Geometry: see drawing. Coordinates: mm, zero at the bounding-box minimum. Coordinates: 2 decimals unless noted, no trailing zeros. Order: outer loops, then holes, each group sorted by start corner. A loop starts at its lowest first (then second) coordinate and runs counter-clockwise, first axis right, second up. Notation, with made-up numbers: (37.5, -29.5) - (45.5, -29.5) arc R22 ccw to (45.5, -14.5) - close; hole circle Ø3 at (30.5, 15.25). An arc over 180 degrees is marked (long way). Use a Markdown table: item, result. Add a question column.
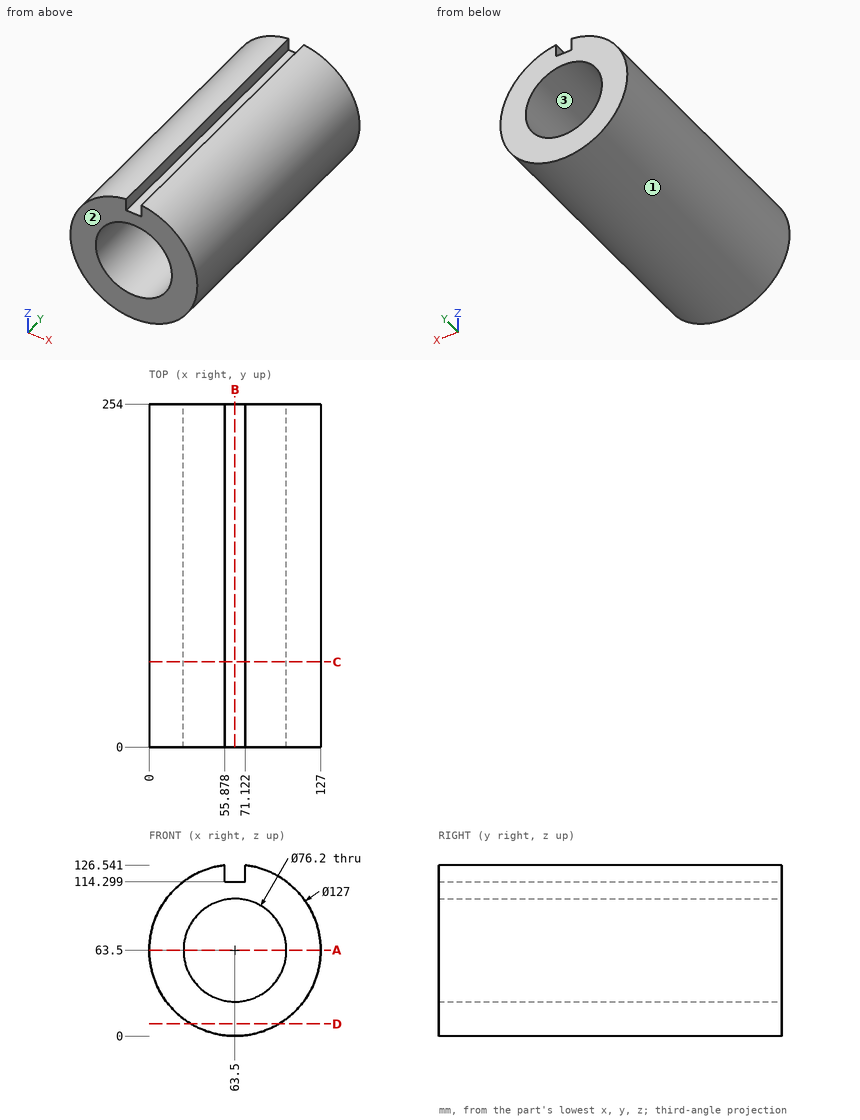
1) Contact query for flat-ended pins moving along their axis: P1, Ø12, axis at y = 118, z = 75, coming from the -X side; P2, Ø12, axis at x = 63.5, y = 142, coming from the +Z side; P3, Ø5, axis at y = 207, z = 84, coming from the +X side. Output: stop coordinate, or through.
2) Pull-direction query (Z, two-part tool) for the marked faces 1, 2 and 3; classes: pulls with the +Z half, pulls with the -Z half, needs draft (parallel to the pull), parting line crosses it, or undercut.
3) Cut plane C-C (y = 63). Return the cut outline in (x, z), and give its area (3 significant figures).
4) Cut plane D-D (z = 9). Return the cut outline in (x, y).
5) Material intervals for L1, parallel to Z at x = 63.5, y = 134; L2, parallel to X at y = 73, z = 63; L3, parallel to X at y = 186, z = 94.5, sorted ascending.
6) Cut plane A-A (z = 63.5). Return the cut outline in (x, y).
7) Cut plane B-B (x = 63.5). Return the cut outline in (y, z).
Computed:
| question | item | result |
|---|---|---|
| 1 | P1 | stops at x = 0.24 |
| 1 | P2 | stops at z = 114.3 |
| 1 | P3 | stops at x = 124.4 |
| 2 | face 1 | parting line crosses it |
| 2 | face 2 | needs draft |
| 2 | face 3 | undercut |
| 3 | outline | (55.88, 114.3) - (55.88, 126.54) arc R63.5 ccw (long way) to (71.12, 126.54) - (71.12, 114.3) - close; hole circle Ø76.2 at (63.5, 63.5) |
| 3 | area | 7,920 mm2 |
| 4 | outline | (30.91, 0) - (96.09, 0) - (96.09, 254) - (30.91, 254) - close |
| 5 | L1 | z = 0 to 25.4, 101.6 to 114.3 |
| 5 | L2 | x = 0 to 25.4, 101.6 to 127 |
| 5 | L3 | x = 8.08 to 41.35, 85.65 to 118.92 |
| 6 | outline | (0, 0) - (25.4, 0) - (25.4, 254) - (0, 254) - close; (101.6, 0) - (127, 0) - (127, 254) - (101.6, 254) - close |
| 7 | outline | (0, 0) - (254, 0) - (254, 25.4) - (0, 25.4) - close; (0, 101.6) - (254, 101.6) - (254, 114.3) - (0, 114.3) - close |
